Build history of the part. All positions in model axes, mm. A direction names the side the tool comes from. Round coordinates to 2 decimals unless told otherwise and drop trailing zeros. Use a Markdown table: item, result.
from build123d import *

# Parameters (mm, degrees)
SKETCH1_R           = 0.95
SKETCH1_W           = 4.2
SKETCH1_H           = 6
SKETCH1_H_2         = 8
BOSS_EXTRUDE1_DEPTH = 2


with BuildPart() as part:
    # Sketch1 → Boss-Extrude1 (new body)
    with BuildSketch(Plane.XY):
        with BuildLine():
            Line((2, 47.74), (4, 47.74))
            Line((4, 47.74), (4, 55.74))
            Line((4, 55.74), (2, 55.74))
            ThreePointArc((2, 55.74), (0.585786438, 56.325786438), (0, 57.74))
            Line((0, 57.74), (0, 68.385))
            ThreePointArc((0, 68.385), (0.585786438, 69.799213562), (2, 70.385))
            Line((2, 70.385), (4, 70.385))
            Line((4, 70.385), (4, 76.385))
            Line((4, 76.385), (2, 76.385))
            ThreePointArc((2, 76.385), (0.585786438, 76.970786438), (0, 78.385))
            Line((0, 78.385), (0, 85.59))
            Line((0, 85.59), (16.2, 85.59))
            Line((16.2, 85.59), (16.2, 78.385))
            ThreePointArc((16.2, 78.385), (15.614213562, 76.970786438), (14.2, 76.385))
            Line((14.2, 76.385), (12.2, 76.385))
            Line((12.2, 76.385), (12.2, 70.385))
            Line((12.2, 70.385), (14.2, 70.385))
            ThreePointArc((14.2, 70.385), (15.614213562, 69.799213562), (16.2, 68.385))
            Line((16.2, 68.385), (16.2, 57.74))
            ThreePointArc((16.2, 57.74), (15.614213562, 56.325786438), (14.2, 55.74))
            Line((14.2, 55.74), (12.2, 55.74))
            Line((12.2, 55.74), (12.2, 47.74))
            Line((12.2, 47.74), (14.2, 47.74))
            ThreePointArc((14.2, 47.74), (15.614213562, 47.154213562), (16.2, 45.74))
            Line((16.2, 45.74), (16.2, 28))
            ThreePointArc((16.2, 28), (15.614213562, 26.585786438), (14.2, 26))
            Line((14.2, 26), (12.2, 26))
            Line((12.2, 26), (12.2, 14))
            Line((12.2, 14), (10.2, 14))
            Line((10.2, 14), (10.2, 26))
            Line((10.2, 26), (6, 26))
            Line((6, 26), (6, 14))
            Line((6, 14), (4, 14))
            Line((4, 14), (4, 26))
            Line((4, 26), (2, 26))
            ThreePointArc((2, 26), (0.585786438, 26.585786438), (0, 28))
            Line((0, 28), (0, 45.74))
            ThreePointArc((0, 45.74), (0.585786438, 47.154213562), (2, 47.74))
        make_face()
        with Locations((13.45, 45.24)):
            Circle(SKETCH1_R, mode=Mode.SUBTRACT)
        with Locations((2.75, 67.885)):
            Circle(SKETCH1_R, mode=Mode.SUBTRACT)
        with Locations((13.45, 58.24)):
            Circle(SKETCH1_R, mode=Mode.SUBTRACT)
        with Locations((13.45, 78.385)):
            Circle(SKETCH1_R, mode=Mode.SUBTRACT)
        with Locations((2.75, 28.5)):
            Circle(SKETCH1_R, mode=Mode.SUBTRACT)
        with Locations((2.75, 78.385)):
            Circle(SKETCH1_R, mode=Mode.SUBTRACT)
        with Locations((2.75, 58.24)):
            Circle(SKETCH1_R, mode=Mode.SUBTRACT)
        with Locations((6, 83.635)):
            Circle(SKETCH1_R, mode=Mode.SUBTRACT)
        with Locations((13.45, 28.5)):
            Circle(SKETCH1_R, mode=Mode.SUBTRACT)
        with Locations((13.45, 67.885)):
            Circle(SKETCH1_R, mode=Mode.SUBTRACT)
        with Locations((10.2, 83.635)):
            Circle(SKETCH1_R, mode=Mode.SUBTRACT)
        with Locations((2.75, 45.24)):
            Circle(SKETCH1_R, mode=Mode.SUBTRACT)
        with Locations((8.1, 73.385)):
            Rectangle(SKETCH1_W, SKETCH1_H, mode=Mode.SUBTRACT)
        with Locations((8.1, 51.74)):
            Rectangle(SKETCH1_W, SKETCH1_H_2, mode=Mode.SUBTRACT)
    extrude(amount=BOSS_EXTRUDE1_DEPTH)


solid = part.part
Q1. Drop flat-ended pins along their axis: pin 1 (1 mm diameter, centred on x = 13, z = 0.5, fed in from -Y); pin 2 (2.5 mm diameter, centred on x = 2.75, y = 78.385, fed in from -Z); pin 3 (1 mm diameter, centred on y = 20, z = 1, fed in from +X); pin 4 (1 mm diameter, centred on y = 75, z = 1, fed in from -X). Give the stop position or say it passes through.
Results found:
| item | result |
|---|---|
| pin 1 | stops at y = 26 |
| pin 2 | stops at z = 0 |
| pin 3 | stops at x = 12.2 |
| pin 4 | stops at x = 4 |
Q2. Cut at A-A, the plane x = 13.45. Count the separate pieces of the cut face and the enclosed holes in it, plus the area to 3 significant figures.
Results found:
| item | result |
|---|---|
| separate pieces | 8 |
| enclosed holes | 0 |
| area | 72.2 mm2 |
Q3. Probe line 1 (Y direction, x = 7.75, z = 0.3) (3 decimals); line 2 (X direction, y = 58.24, z = 1.2); line 3 (X direction, y = 21, z = 1.1). List the from-to ranges inside material, lowest first.
Results found:
| item | result |
|---|---|
| line 1 | y = 26 to 47.74, 55.74 to 70.385, 76.385 to 85.59 |
| line 2 | x = 0 to 1.8, 3.7 to 12.5, 14.4 to 16.2 |
| line 3 | x = 4 to 6, 10.2 to 12.2 |
Q4. Pull direction X, two halves, no side cores. Call faces 5 (the face through (16.2, 37, 1)), 6 (the face through (0.6, 56.31, 0.99)), 7 (the face through (8, 47.74, 1)): pulls with the +X half, pulls with the -X half, needs draft (parallel to the pull), parting line crosses it, or undercut.
Results found:
| item | result |
|---|---|
| face 5 | pulls with the +X half |
| face 6 | pulls with the -X half |
| face 7 | undercut |
Q5. Which spindle directions (+Z, -Z, +X, -X, +Y, -Y) get a long thin tool onto all of the face, cutting with end or side? Do faces 1 (the face through (13, 70.385, 1)), 2 (the face through (0.57, 69.784, 0.986)), 3 (the face through (12.2, 20, 1)), 4 (the face through (10.2, 20, 1)). Say none if no direction does.
Results found:
| item | result |
|---|---|
| face 1 | +Z, -Z, +X |
| face 2 | +Z, -Z, -X |
| face 3 | +Z, -Z, +X, -Y |
| face 4 | +Z, -Z, -Y |
